Check sheet for the drawn part. Datum: minimum x, y, z corner. Units: mm. A direction names the side the tool comes from. Give positions to 0.01 mm unless a question says otherwise; leave off trailing zeros. Order: outer loops, then holes, each group sorted by start corner. A loop starts at its lowest first (then second) coordinate and runs counter-clockwise, first axis right, second up. Notation, with made-up numbers: M -17,19.5 L 2,19.5 A8 cw 2,26.5 Z; hole C 26,39 d5. An arc over 180 degrees is marked long. One line per question, with ' | ' between items. Start each with the question number.
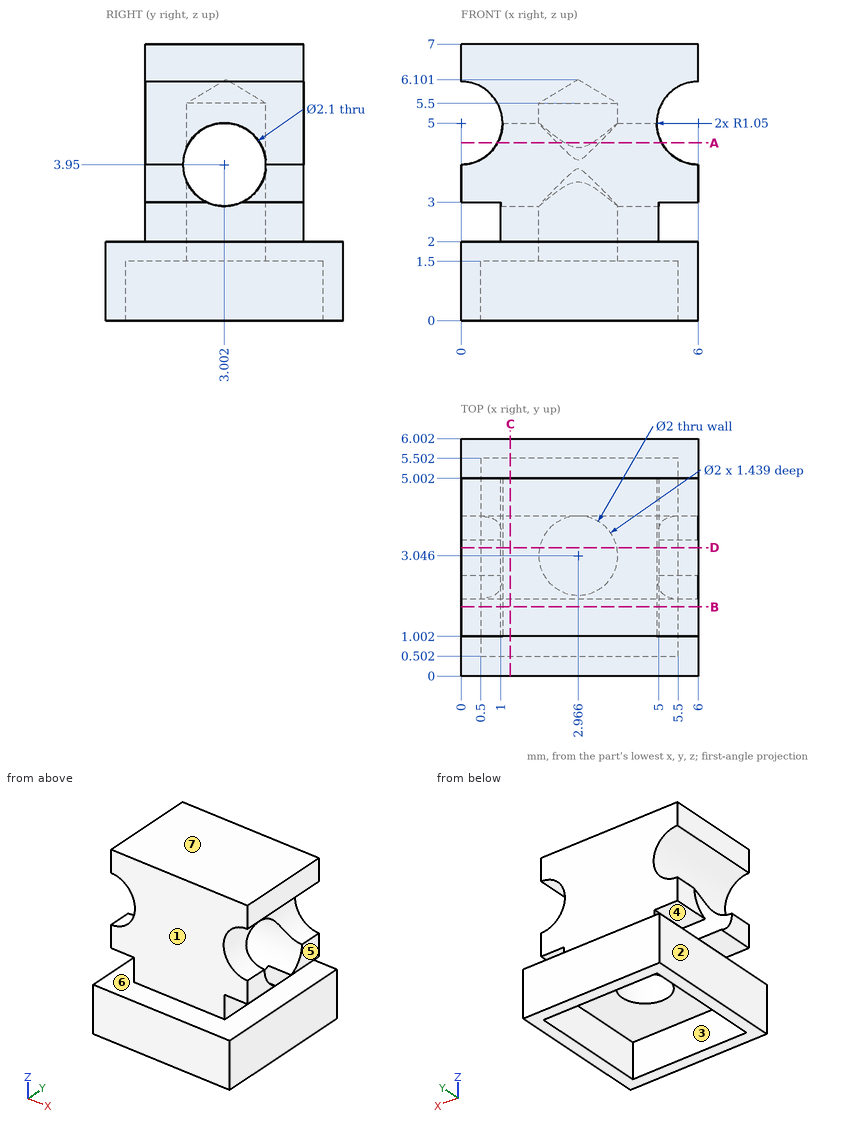
Item 1: Scan lines: probe 1 along Y at (x, z) = (1, 4); probe 2 along X at (y, z) = (3.5, 0.75). Record each from-to range of solid material in increasing order. Write a range as [from, to].
Item 2: Section check D-D, the plane y = 3.25. State how many separate pieces and enclosed holes the cut face has.
Item 3: Go/stop test with flat-tipped pins: P1, Ø0.8, axis at y = 2.5, z = 2.5, coming from the +X side; P2, Ø1.5, axis at x = 3.5, y = 2.5, coming from the -Z side; P3, Ø1.5, axis at x = 1, z = 3.5, coming from the +Y side. Record where each tip stops, or that it passes through.
Item 4: Set-up check for the marked faces 1, 2, 3 and 4: record each of +Z, -Z, +X, -X, +Y, -Y from which the full face is reachable in a straight line by a thin tool's end or side.
Item 5: Section check B-B, the plane y = 1.75. Record the cut outline in (x, z).
Item 6: Section check A-A, the plane z = 4.5. Record the cut outline in (x, y).
Item 7: Section check C-C, the plane x = 1.25. Record the cut outline in (y, z).
Item 8: Draft check along Z on the marked faces 5, 6 and 7. Enter one of: released by +Z, released by -Z, zero draft, split by the parting line, or undercut.
Reported:
1) probe 1: y = [1, 1.95], [4.05, 5] | probe 2: x = [0, 0.5], [5.5, 6]
2) separate pieces: 3 | enclosed holes: 0
3) P1: stops at x = 5 | P2: stops at z = 1.5 | P3: stops at y = 5
4) face 1: +Z, +X, -X, -Y | face 2: +Z, -Z, -X, +Y, -Y | face 3: -Z | face 4: -X, +Y, -Y
5) outline: M 0,0 L 0.5,0 L 0.5,1.5 L 5.5,1.5 L 5.5,0 L 6,0 L 6,2 L 5,2 L 5,3 L 6,3 L 6,3.95 A1.05 cw 6,6.05 L 6,7 L 0,7 L 0,6.05 A1.05 cw 0,3.95 L 0,3 L 1,3 L 1,2 L 0,2 Z
6) outline: M 0.92,1 L 5.08,1 L 5.08,2.11 L 3.31,2.11 A1 cw 2.62,2.11 L 0.92,2.11 Z; M 0.92,3.9 L 2.44,3.9 A1 cw 3.49,3.9 L 5.08,3.9 L 5.08,5 L 0.92,5 Z
7) outline: M 0,0 L 0.5,0 L 0.5,1.5 L 5.5,1.5 L 5.5,0 L 6,0 L 6,2 L 5,2 L 5,7 L 1,7 L 1,2 L 0,2 Z; hole C 3,3.95 d2.1
8) face 5: zero draft | face 6: undercut | face 7: released by +Z
